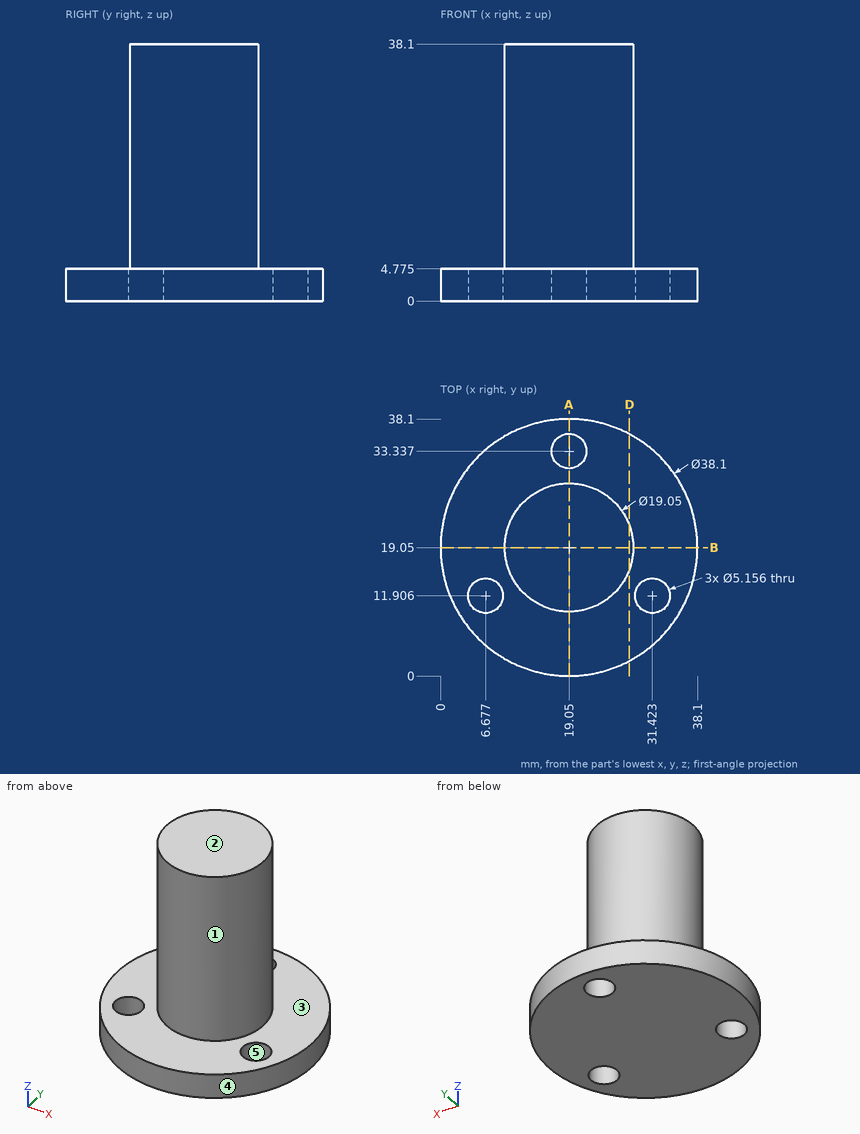
The figure shows three views and two pictorial views of one solid part (mm, origin at its lowest corner). Answer the questions. A direction names the side the tool comes from. Round coordinates to 2 decimals unless told otherwise and drop trailing zeros. Write each loop counter-clockwise with the first axis right and the second up, starting at its lowest first coordinate (ties: lowest second). Pieces come first, ordered by that corner, then holes. Notation, with made-up numbers: M 27,5.25 L 75,5.25 A26 ccw 75,41.25 Z; hole C -15.5,-24.5 d4. An arc over 180 degrees is marked long. Use a Markdown table: item, result.
1) The part is cut by section B-B on y = 19.05. Give the vertices of the cut face in (x, z) (1 decimal).
Taken from the geometry:
| item | result |
|---|---|
| outline | M 0,0 L 38.1,0 L 38.1,4.8 L 28.6,4.8 L 28.6,38.1 L 9.5,38.1 L 9.5,4.8 L 0,4.8 Z |
2) The part is cut by section D-D on x = 28. Give the vertices of the cut face in (y, z) (1 decimal).
Taken from the geometry:
| item | result |
|---|---|
| outline | M 2.2,0 L 35.9,0 L 35.9,4.8 L 22.3,4.8 L 22.3,38.1 L 15.8,38.1 L 15.8,4.8 L 2.2,4.8 Z |
3) Which of the six approach directions +Z, -Z, +X, -X, +Y, -Y give full straight-line access (tool end or side, diameter ignored) to the marked faces 1 and 2?
Taken from the geometry:
| item | result |
|---|---|
| face 1 | +Z |
| face 2 | +Z, +X, -X, +Y, -Y |
4) The part is cut by section A-A on x = 19.05. Give the vertices of the cut face in (y, z) (1 decimal).
Taken from the geometry:
| item | result |
|---|---|
| outline | M 0,0 L 30.8,0 L 30.8,4.8 L 28.6,4.8 L 28.6,38.1 L 9.5,38.1 L 9.5,4.8 L 0,4.8 Z; M 35.9,0 L 38.1,0 L 38.1,4.8 L 35.9,4.8 Z |
5) Flat-ended cylindrical pins translate along their axes: pin 1 (6.5 mm diameter, centred on x = 31.42, y = 11.91, fed in from +Z) (1 decimal); pin 2 (2 mm diameter, centred on y = 18, z = 9, fed in from -X) (1 decimal); pin 3 (12 mm diameter, centred on x = 21.5, z = 15.5, fed in from +Y) (1 decimal). Find the tip coordinate at first contact, or state that the pin passes through.
Taken from the geometry:
| item | result |
|---|---|
| pin 1 | stops at z = 4.8 |
| pin 2 | stops at x = 9.5 |
| pin 3 | stops at y = 28.6 |
6) Determine the mould class of the marked faces 3, 4 and 5 for opening direction X: pulls with the +X half, pulls with the -X half, needs draft (parallel to the pull), parting line crosses it, or undercut.
Taken from the geometry:
| item | result |
|---|---|
| face 3 | needs draft |
| face 4 | parting line crosses it |
| face 5 | undercut |
7) Consider line 1 (Y direction, x = 19.05, z = 2.25) (1 decimal); line 2 (Z direction, x = 10.5, y = 28.5) (1 decimal); line 3 (Y direction, x = 12, z = 33) (1 decimal). Determine where each line is inside the solid, lowest interval first. Write a range as [from, to].
Taken from the geometry:
| item | result |
|---|---|
| line 1 | y = [0, 30.8], [35.9, 38.1] |
| line 2 | z = [0, 4.8] |
| line 3 | y = [12.6, 25.5] |
